Geometry check sheet. Reference: the model listing, model coordinates, mm. Give positions to 0.01 mm unless a question says otherwise; leave off trailing zeros. Write each loop counter-clockwise with the first axis right and the second up, starting at its lowest first coordinate (ties: lowest second). Pieces come first, ordered by that corner, then holes. Notation, with made-up numbers: (47.25, -14.5) - (104.25, -14.5) arc R8 cw to (104.25, -7.5) - close; hole circle Ø9 at (76, 76.25). An arc over 180 degrees is marked (long way). Write item = value, one per line. Start each with the question number.
(1) Depth check by flat-ended pin: pin 1 Ø1.5 at (x, y) = (45, -20) entering from +Z; pin 2 Ø2 at (x, y) = (31, -19) entering from -Z. Enter the tip coordinate at first touch or a pass-through.
(2) Section check A-A, the plane y = -19.5. Give the number of separate pieces and of enclosed holes in the cut face, plus the area to 3 significant figures.
(3) Section check C-C, the plane x = 34.5. Enter the section's corners in (y, z).
(4) Thickness scan on L1, parallel to X at y = -20.75, z = 90.55; L2, parallel to X at y = -20.5, z = 90.6; L3, parallel to Z at x = 24.5, y = -21.5. Record the ranges inside material, lowest first.
```python
from build123d import *

# Parameters (mm, degrees)
SKETCH1_R           = 1.595
SKETCH1_R_2         = 1.5
BOSS_EXTRUDE1_DEPTH = 1


with BuildPart() as part:
    # Sketch1 → Boss-Extrude1 (new body)
    with BuildSketch(Plane(origin=(0.276968936, -0.030405965, 89.917439906), x_dir=(0.999995256, 1.042e-06, -0.003080243), z_dir=(0.003080243, -0.000338153, 0.999995199))):
        with BuildLine():
            Line((29.351122384, -23.602694705), (47.163406232, -23.602694705))
            Line((47.163406232, -23.602694705), (47.163406232, -17.90355794))
            Line((47.163406232, -17.90355794), (29.351122384, -17.90355794))
            ThreePointArc((29.351122384, -17.90355794), (23.163406232, -20.753126322), (29.351122384, -23.602694705))
        make_face()
        with Locations((26.913406232, -20.753126322)):
            Circle(SKETCH1_R, mode=Mode.SUBTRACT)
        with Locations((44.663406232, -20.753126322)):
            Circle(SKETCH1_R_2, mode=Mode.SUBTRACT)
    extrude(amount=BOSS_EXTRUDE1_DEPTH)


solid = part.part
```
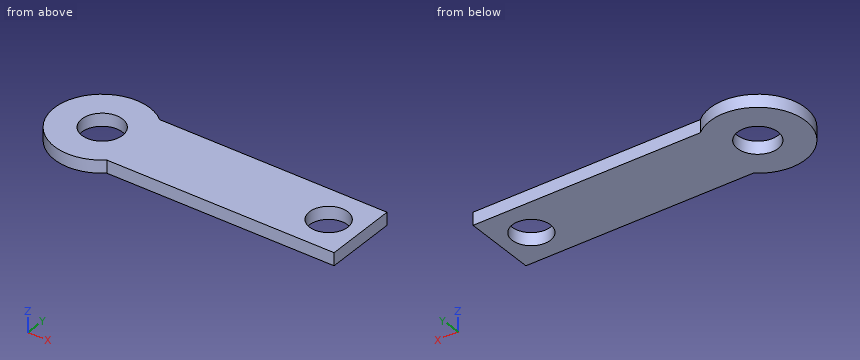
Model answer:
q1.pin_1 = 90.77
q1.pin_2 = 89.81
q2.separate_pieces = 3
q2.enclosed_holes = 0
q2.area = 20.3 mm²
q3.outline = (-23.63, 89.8) - (-17.93, 89.81) - (-17.93, 90.81) - (-23.63, 90.8) - close
q4.L1 = 23.44 to 25.6, 28.79 to 43.44, 46.44 to 47.44
q4.L2 = 23.45 to 25.62, 28.76 to 43.47, 46.42 to 47.44
q4.L3 = 89.84 to 90.84
